```python
from build123d import *

# Parameters (mm, degrees)
F0_W     = 30
F0_H     = 30
F1_DEPTH = 7
F3_D     = 3.4
F5_DEPTH = 30
F6_R     = 5


with BuildPart() as f1:
    # F0 (on Top) → F1 (new body)
    with BuildSketch(Plane.XY):
        Rectangle(F0_W, F0_H)
    extrude(amount=F1_DEPTH)

    # F3 (through all)
    with Locations(Plane.XY.offset(7)):
        with Locations((-11, 0), (11, 0)):
            Hole(F3_D / 2)

    # F4 (on face) → F5 (cut, through all)
    with BuildSketch(Plane.XZ.offset(15)):
        with BuildLine():
            Line((-5, 0), (5, 0))
            ThreePointArc((5, 0), (0, 5), (-5, 0))
        make_face()
    extrude(amount=-F5_DEPTH, mode=Mode.SUBTRACT)

    # F6
    f6_edges = [f1.edges().sort_by_distance(p)[0] for p in [
        (15, -15, 3.5),
        (-15, -15, 3.5),
        (15, 15, 3.5),
        (-15, 15, 3.5),
    ]]
    fillet(f6_edges, radius=F6_R)


solid = f1.part
```
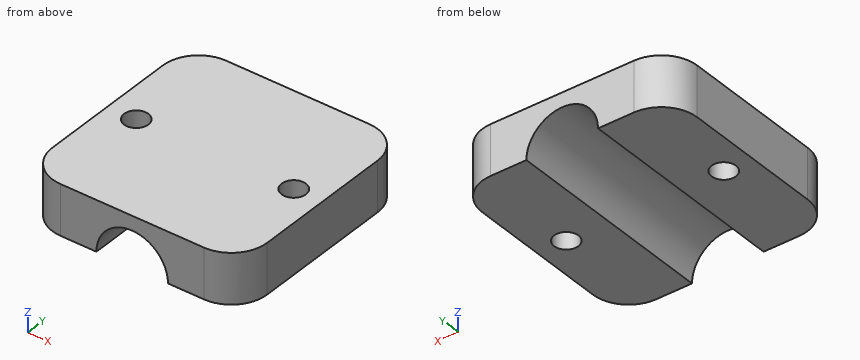
Geometry: final body of the model. Coordinates: model frame, mm. Round coordinates to 2 decimals unless told otherwise and drop trailing zeros. Write each loop counter-clockwise with the first axis right and the second up, starting at its lowest first coordinate (ties: lowest second). Pieces come first, ordered by that corner, then holes. Notation, with made-up numbers: M -30.75,70.25 L 6.25,70.25 A30 ccw 6.25,98.25 Z; hole C 54,10.25 d4. An arc over 180 degrees is marked long. Answer in a Markdown table with one row per item. Add a question column.
(1) Cut plane D-D, the plane z = 5.75. Return the cut outline in (x, y).
(2) Cut plane A-A, the plane z = 3.5. Return the cut outline in (x, y), then the cut area to 3 significant figures.
(3) Ray query, L1, parallel to Y at x = -11, z = 5; L2, parallel to X at y = -13.5, z = 4; L3, parallel to X at y = -6.75, z = 3.5. Return the intervals inside material, ascending.
(4) Cut plane B-B, the plane y = 0. Return the cut outline in (x, z), then the cut area to 3 significant figures.
(5) Cut plane C-C, the plane x = 11. Return the cut outline in (y, z), then the cut area to 3 significant figures.
Established:
| question | item | result |
|---|---|---|
| 1 | outline | M -15,-10 A5 ccw -10,-15 L 10,-15 A5 ccw 15,-10 L 15,10 A5 ccw 10,15 L -10,15 A5 ccw -15,10 Z; hole C -11,0 d3.4; hole C 11,0 d3.4 |
| 2 | outline | M -15,-10 A5 ccw -10,-15 L -3.57,-15 L -3.57,15 L -10,15 A5 ccw -15,10 Z; M 3.57,-15 L 10,-15 A5 ccw 15,-10 L 15,10 A5 ccw 10,15 L 3.57,15 Z; hole C -11,0 d3.4; hole C 11,0 d3.4 |
| 2 | area | 646 mm² |
| 3 | L1 | -14.9 to -1.7, 1.7 to 14.9 |
| 3 | L2 | -13.57 to -3, 3 to 13.57 |
| 3 | L3 | -15 to -3.57, 3.57 to 15 |
| 4 | outline | M -15,0 L -12.7,0 L -12.7,7 L -15,7 Z; M -9.3,0 L -5,0 A5 cw 5,0 L 9.3,0 L 9.3,7 L -9.3,7 Z; M 12.7,0 L 15,0 L 15,7 L 12.7,7 Z |
| 4 | area | 123 mm² |
| 5 | outline | M -14.9,0 L -1.7,0 L -1.7,7 L -14.9,7 Z; M 1.7,0 L 14.9,0 L 14.9,7 L 1.7,7 Z |
| 5 | area | 185 mm² |
